Geometry check sheet. Reference: the model listing, model coordinates, mm. A direction names the side the tool comes from. Give positions to 0.01 mm unless a question says otherwise; leave off trailing zeros. Write each loop counter-clockwise with the first axis right and the second up, starting at its lowest first coordinate (ties: lowest second). Pieces come first, ordered by that corner, then holes. Notation, with made-up numbers: M 54,51 L 98,51 A18 ccw 98,60 Z; hole C 52.25,32 d1. An arc over 180 degrees is marked long. Use one line per item in the form item = value. Start each with the question number.
```python
from build123d import *

# Parameters (mm, degrees)
SKETCH1_R           = 2.25
BOSS_EXTRUDE1_DEPTH = 3
CIRPATTERN1_COUNT   = 2
CIRPATTERN1_ANGLE   = 90
FILLET1_R           = 3


with BuildPart() as part:
    # Sketch1 → Boss-Extrude1 (new body)
    with BuildSketch(Plane.XY):
        with BuildLine():
            Line((-7.75, 6.125), (-7.75, -6.125))
            Line((-7.75, -6.125), (7.75, -6.125))
            Line((7.75, -6.125), (7.75, 6.125))
            ThreePointArc((7.75, 6.125), (0, 13.875), (-7.75, 6.125))
        make_face()
        with Locations((0, 5.875)):
            Circle(SKETCH1_R, mode=Mode.SUBTRACT)
    boss_extrude1 = extrude(amount=BOSS_EXTRUDE1_DEPTH)

    # CirPattern1: Boss-Extrude1 ×2 about axis
    cirpattern1_axis = Axis((-8.525, -4.625, 1.5), (1, 0, 0))
    for i in range(1, CIRPATTERN1_COUNT):
        add(boss_extrude1.rotate(cirpattern1_axis, i * CIRPATTERN1_ANGLE / (CIRPATTERN1_COUNT - 1)))

    # Fillet1
    fillet1_edges = [part.edges().sort_by_distance(p)[0] for p in [
        (0, -6.125, 0),
    ]]
    fillet(fillet1_edges, radius=FILLET1_R)


solid = part.part
```
(1) Sectioned sample at D-D, the plane y = 2.5. Record the boundary of the cut face in (x, z), plus the area to 3 significant figures.
(2) Tool access check on faces 1 (the flat face through (2, -3.125, 10)), 2 (the cylindrical face through (0, -5, 20)). Record the directions out of +Z, -Z, +X, -X, +Y, -Y that give a thin tool (end or side, any length) a straight path to the whole face; none if there is none.
(3) Sectioned sample at C-C, the plane x = 5.25. Record the boundary of the cut face in (y, z) (3 decimals), plus the area to 3 significant figures.
(4) Depth check by flat-ended pin: pin 1 (2 mm diameter, centred on y = -3, z = 10.5, fed in from +X); pin 2 (3.5 mm diameter, centred on x = 0, z = 12, fed in from -Y); pin 3 (6 mm diameter, centred on x = 0.5, y = 2.5, fed in from +Z); pin 4 (4 mm diameter, centred on x = -3, z = 12.5, fed in from +Y) (3 decimals). Enter the tip coordinate at first touch or a pass-through.
(5) Sectioned sample at A-A, the plane x = 0. Record the boundary of the cut face in (y, z) (3 decimals).
(6) Thickness scan on probe 1 along Z at (x, y) = (4.75, 1.75); probe 2 along Z at (x, y) = (0, -4.6); probe 3 along Y at (x, z) = (-2, 17.5) (3 decimals). Record the ranges inside material, lowest first. Write a range as [from, to].
(7) Draft check along Y on faces 3 (the cylindrical face through (0.17, 13.873, 1.479)), 4 (the cylindrical face through (1.21, 7.77, 1.48)), 5 (the cylindrical face through (0.109, -5.223, 0.855)), 6 (the flat face through (7.75, -1, 2)). Enter one of: released by +Y, released by -Y, zero draft, split by the parting line, or undercut.
(8) Sectioned sample at B-B, the plane z = 1.5. Record the boundary of the cut face in (x, y) (3 decimals).
Numbers:
q1.outline = M -7.75,0 L 7.75,0 L 7.75,3 L -7.75,3 Z
q1.area = 46.5 mm2
q2.face_1 = +Z, +X, -X, +Y
q2.face_2 = +Z, +Y, -Y
q3.outline = M -6.125,3 A3 ccw -3.125,0 L 11.826,0 L 11.826,3 L -3.125,3 L -3.125,17.951 L -6.125,17.951 Z
q3.area = 96.8 mm2
q4.pin_1 = 7.75
q4.pin_2 = through
q4.pin_3 = 3
q4.pin_4 = -3.125
q5.outline = M -6.125,3 A3 ccw -3.125,0 L 3.625,0 L 3.625,3 L -3.125,3 L -3.125,9.75 L -6.125,9.75 Z; M -6.125,14.25 L -3.125,14.25 L -3.125,20 L -6.125,20 Z; M 8.125,0 L 13.875,0 L 13.875,3 L 8.125,3 Z
q6.probe_1 = [0, 3]
q6.probe_2 = [0.39, 9.75], [14.25, 20]
q6.probe_3 = [-6.125, -3.125]
q7.face_3 = released by +Y
q7.face_4 = undercut
q7.face_5 = released by -Y
q7.face_6 = zero draft
q8.outline = M -7.75,-5.723 L 7.75,-5.723 L 7.75,6.125 A7.75 ccw -7.75,6.125 Z; hole C 0,5.875 d4.5
